Part model, mm, in its own coordinate system. Coordinates: 2 decimals unless noted, no trailing zeros. Loops run counter-clockwise (first coordinate to the right, second up) from the corner with the lowest first, then second, coordinate; pieces in that order, holes last. Notation, with made-up numbers: (0.25, -11) -> (53.25, -11) arc R22 cw to (53.25, 28) -> close; hole circle Ø1 at (0, 8.25). An arc over 180 degrees is marked (long way). Use one line per item in the form item = value. Start each with the question number.
(1) Pin check, flat tip, straight feed: P1, Ø5.5, axis at x = 20, y = 20, coming from the -Z side. Stop position of the tip, or through.
(2) Band-saw the part on D-D on z = 1.85. Count the separate pieces of the cut face and the enclosed holes in it, then the cut area to 3 significant figures.
(3) Band-saw the part on B-B on x = 0. Give the cut face in (y, z).
(4) Band-saw the part on C-C on y = 0. Give the cut face in (x, z).
(5) Drill centre lines: L1, parallel to Y at x = 20, z = 1.45; L2, parallel to Y at x = 0, z = 4.05; L3, parallel to X at y = -17, z = 2.6. Where is each one in solid material? Low to high. Write a range as [from, to].
(6) Band-saw the part on A-A on y = -52.5. Give the cut face in (x, z), then the cut area to 3 significant figures.
```python
from build123d import *

# Parameters (mm, degrees)
F0_W             = 110
F0_H             = 135
F1_DEPTH         = 5
F2_R             = 3.5
F2_R_2           = 5.5
F3_DEPTH         = 25
F5_DEPTH         = 25
F5_COPIES2_COUNT = 2
F5_COPIES2_PITCH = 132.003788
F6_R             = 5


# Not quite as in the source:
# - a pattern or mirror of a feature is missing from the dataset's text; its kind, count and spacing are read off the source's solid


with BuildPart() as f1:
    # F0 (on Top) → F1 (new body)
    with BuildSketch(Plane.XY):
        Rectangle(F0_W, F0_H)
    extrude(amount=F1_DEPTH)

    # F2 (on face) → F3 (cut)
    with BuildSketch(Plane.XY.offset(5)):
        with Locations((-20, 20)):
            Circle(F2_R)
        with Locations((20, 20)):
            Circle(F2_R)
        with Locations((20, -20)):
            Circle(F2_R)
        with Locations((-20, -20)):
            Circle(F2_R)
        Circle(F2_R_2)
    extrude(amount=-F3_DEPTH, mode=Mode.SUBTRACT)

    # F4 (on face) → F5 (cut)
    with BuildSketch(Plane.XY.offset(5)):
        with BuildLine():
            ThreePointArc((-41.5, 58.5), (-47.5, 52.5), (-41.5, 46.5))
            Line((-41.5, 46.5), (-38.5, 46.5))
            ThreePointArc((-38.5, 46.5), (-32.5, 52.5), (-38.5, 58.5))
            Line((-38.5, 58.5), (-41.5, 58.5))
        make_face()
    f5 = extrude(amount=-F5_DEPTH, mode=Mode.SUBTRACT)

    # F5_copies: F5 across plane
    add(f5.mirror(Plane(origin=(0, 0, 0), x_dir=(0, 0, -1), z_dir=(0, -1, 0))), mode=Mode.SUBTRACT)

    # F5_copies1: F5 across plane
    add(f5.mirror(Plane(origin=(0, 0, 0), x_dir=(0, 0, 1), z_dir=(1, 0, 0))), mode=Mode.SUBTRACT)

    # F5_copies2: F5 ×2
    with Locations(*[Vector(0.6060432153, -0.79543172, 0) * (i * F5_COPIES2_PITCH) for i in range(1, F5_COPIES2_COUNT)]):
        add(f5, mode=Mode.SUBTRACT)

    # F6
    f6_edges = [f1.edges().sort_by_distance(p)[0] for p in [
        (-55, 67.5, 2.5),
        (55, 67.5, 2.5),
        (55, -67.5, 2.5),
        (-55, -67.5, 2.5),
    ]]
    fillet(f6_edges, radius=F6_R)


solid = f1.part
```
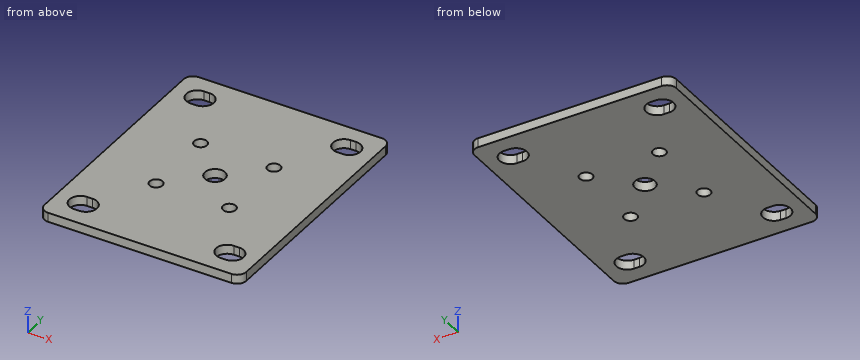
A:
q1.P1 = through
q2.separate_pieces = 1
q2.enclosed_holes = 9
q2.area = 14,000 mm²
q3.outline = (-67.5, 0) -> (-5.5, 0) -> (-5.5, 5) -> (-67.5, 5) -> close; (5.5, 0) -> (67.5, 0) -> (67.5, 5) -> (5.5, 5) -> close
q4.outline = (-55, 0) -> (-5.5, 0) -> (-5.5, 5) -> (-55, 5) -> close; (5.5, 0) -> (55, 0) -> (55, 5) -> (5.5, 5) -> close
q5.L1 = [-67.5, -23.5], [-16.5, 16.5], [23.5, 67.5]
q5.L2 = [-67.5, -5.5], [5.5, 67.5]
q5.L3 = [-55, -21.8], [-18.2, 18.2], [21.8, 55]
q6.outline = (-55, 0) -> (-47.5, 0) -> (-47.5, 5) -> (-55, 5) -> close; (-32.5, 0) -> (32.5, 0) -> (32.5, 5) -> (-32.5, 5) -> close; (47.5, 0) -> (55, 0) -> (55, 5) -> (47.5, 5) -> close
q6.area = 400 mm²
